Autodesk Inventor part; units mm, degrees
ref_plane "YZ Plane" through (0, 0, 0) normal (1, 0, 0) x (0, 1, 0)
ref_plane "XZ Plane" through (0, 0, 0) normal (0, 1, 0) x (-1, 0, 0)
ref_plane "XY Plane" through (0, 0, 0) normal (0, 0, 1) x (1, 0, 0)
sketch "Sketch1" plane through (0, 0, 0) normal (0, 0, 1) x (1, 0, 0)
  circle A0 centre (0, 0) radius 35
  circle A1 centre (0, 120) radius 35
  arc A2 (-50, 0) -> (50, 0) centre (0, 0) ccw
  arc A3 (50, 120) -> (-50, 120) centre (0, 120) ccw
  line L0 (-50, 0) -> (-50, 120)
  line L1 (50, 0) -> (50, 120)
  line L2 (0, 35) -> (0, 85)
  dimension "d0" = 70
  dimension "d1" = 70
  dimension "d3" = 15
  dimension "d4" = 15
  dimension "d7" = 50
extrude "Extrusion1" add sketch "Sketch1" along normal blind 35
sketch "Sketch2" plane through (50, 0, 0) normal (1, 0, 0) x (0, 0, -1)
  line L0 (-35, 170) -> (0, 170)
  line L1 (0, 170) -> (0, -50)
  line L2 (0, -50) -> (-35, -50)
  line L3 (-35, -50) -> (-35, 170)
  line L4 (-2.5, -47.5) -> (-2.5, 167.5)
  line L5 (-2.5, 167.5) -> (-32.5, 167.5)
  line L6 (-32.5, 167.5) -> (-32.5, -47.5)
  line L7 (-32.5, -47.5) -> (-32.5, -50)
  line L8 (-2.5, -47.5) -> (-2.5, -50)
  dimension "d8" = 220
  dimension "d9" = 2.5
extrude "Extrusion2" cut sketch "Sketch2" against normal blind 300 contours L7 L6 L5 L4 L8 L2
properties part number "sambungan leaf spring 1" material "Steel, Mild"
CAD build for the part. Positions are in the model's coordinates, mm. A direction names the side the tool comes from. Round coordinates to 2 decimals unless told otherwise and drop trailing zeros. Write each loop counter-clockwise with the first axis right and the second up, starting at its lowest first coordinate (ties: lowest second). Pieces come first, ordered by that corner, then holes.
(1) Slice it at D-D, the plane y = 125.5. Write the cut outline in (x, z).
(2) Drop flat-ended pins along their axis: P1, Ø10, axis at y = -15.5, z = 25, coming from the +X side; P2, Ø12, axis at x = 14.5, z = 19.5, coming from the +Y side; P3, Ø3, axis at x = -1.5, z = 8, coming from the +Y side; P4, Ø9, axis at x = -8, z = 18, coming from the -Y side. Give the stop position or say it passes through.
(3) Slice it at B-B, the plane y = 43.5. Write the cut outline in (x, z).
(4) Mould opens along Z. For faces 3 (the face through (-1, 62, 0)), 4 (the face through (-7.587, 154.168, 33.732)), 5 (the face through (1, 57, 2.5)) say: pulls with the +Z half, pulls with the -Z half, needs draft (parallel to the pull), parting line crosses it, or undercut.
(5) Probe line 1 along Y through (x, z) = (0, 33); line 2 along Z through (x, y) = (-2, 81); line 3 along X through (y, z) = (0, 1). List the from-to ranges inside material, lowest first.
(6) Slice it at C-C, the plane x = -22.5. Write the cut outline in (y, z), and give its area (3 significant figures).
(7) Slice it at A-A, the plane x = 0. Write the cut outline in (y, z), and give its area (3 significant figures).
(8) 3-axis set-ups, long thin cutter, end or side, ignore diameter. For faces 1 (the face through (1.099, -49.988, 1.232)), 2 (the face through (1, 60, 32.5)): which of +Z, -Z, +X, -X, +Y, -Y reach the whole face in a straight line?
From the geometry:
1. outline: (-49.7, 0) - (-34.57, 0) - (-34.57, 2.5) - (-49.7, 2.5) - close; (-49.7, 32.5) - (-34.57, 32.5) - (-34.57, 35) - (-49.7, 35) - close; (34.57, 0) - (49.7, 0) - (49.7, 2.5) - (34.57, 2.5) - close; (34.57, 32.5) - (49.7, 32.5) - (49.7, 35) - (34.57, 35) - close
2. P1: passes through
2. P2: stops at y = 169.27
2. P3: stops at y = 170
2. P4: stops at y = 167.5
3. outline: (-50, 0) - (50, 0) - (50, 2.5) - (-50, 2.5) - close; (-50, 32.5) - (50, 32.5) - (50, 35) - (-50, 35) - close
4. face 3: pulls with the -Z half
4. face 4: needs draft
4. face 5: undercut
5. line 1: y = -50 to -35, 35 to 85, 155 to 170
5. line 2: z = 0 to 2.5, 32.5 to 35
5. line 3: x = -50 to -35, 35 to 50
6. outline: (-44.65, 0) - (-26.81, 0) - (-26.81, 2.5) - (-44.65, 2.5) - close; (-44.65, 32.5) - (-26.81, 32.5) - (-26.81, 35) - (-44.65, 35) - close; (26.81, 0) - (93.19, 0) - (93.19, 2.5) - (26.81, 2.5) - close; (26.81, 32.5) - (93.19, 32.5) - (93.19, 35) - (26.81, 35) - close; (146.81, 0) - (164.65, 0) - (164.65, 2.5) - (146.81, 2.5) - close; (146.81, 32.5) - (164.65, 32.5) - (164.65, 35) - (146.81, 35) - close
6. area: 510 mm2
7. outline: (-50, 0) - (-35, 0) - (-35, 2.5) - (-50, 2.5) - close; (-50, 32.5) - (-35, 32.5) - (-35, 35) - (-50, 35) - close; (35, 0) - (85, 0) - (85, 2.5) - (35, 2.5) - close; (35, 32.5) - (85, 32.5) - (85, 35) - (35, 35) - close; (155, 0) - (170, 0) - (170, 35) - (155, 35) - (155, 32.5) - (167.5, 32.5) - (167.5, 2.5) - (155, 2.5) - close
7. area: 475 mm2
8. face 1: +Z, -Z, -Y
8. face 2: +X, -X, -Y
